```python
from build123d import *


with BuildPart() as part:
    # Sketch1 → Revolve1 (revolve)
    with BuildSketch(Plane(origin=(0, 0, 0), x_dir=(0, -1, 0), z_dir=(0, 0, -1)), mode=Mode.PRIVATE) as revolve1_sk:
        with BuildLine():
            Line((0, 1.5), (0, 12.78))
            Line((0, 12.78), (-0.18, 12.78))
            Line((-0.18, 12.78), (-0.18, 7.65))
            Line((-0.18, 7.65), (-0.5, 7.65))
            Line((-0.5, 7.65), (-0.5, 6.8))
            ThreePointArc((-0.5, 6.8), (-0.646446609, 6.446446609), (-1, 6.3))
            Line((-1, 6.3), (-3.7, 6.3))
            Line((-3.7, 6.3), (-4.2, 5.8))
            Line((-4.2, 5.8), (-4.2, 5.1))
            Line((-4.2, 5.1), (-5.4, 5.1))
            Line((-5.4, 5.1), (-5.9, 4.6))
            Line((-5.9, 4.6), (-5.9, 2))
            Line((-5.9, 2), (-5.4, 1.5))
            Line((-5.4, 1.5), (0, 1.5))
        make_face()
    revolve(revolve1_sk.sketch.rotate(Axis((0, 0, 0), (0, 1, 0)), 180), axis=Axis((0, 0, 0), (0, 1, 0)))


solid = part.part
```
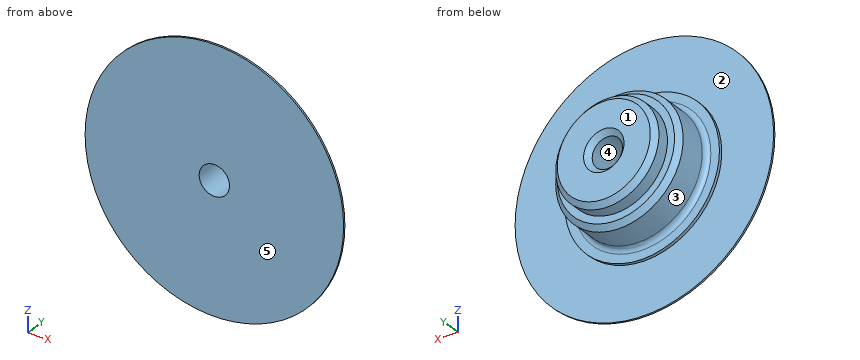
Could you check a few things on this model? Use its own coordinates, in mm. Face numbers are marked on the shaded views. A direction names the side the tool comes from. Round coordinates to 2 decimals unless told otherwise and drop trailing zeros. Order: outer loops, then holes, each group sorted by start corner. A loop starts at its lowest first (then second) coordinate and runs counter-clockwise, first axis right, second up. Notation, with made-up numbers: M 77.5,4 L 135.5,4 A23 cw 135.5,16 Z; hole C -34,-3.5 d10. An arc over 180 degrees is marked long. One line per question, with ' | ' between items. Start each with the question number.
(1) Suppose I cut it at B-B on x = 0. List the corners of the cut face in (y, z) for me, then the cut area to 3 significant figures.
(2) For P1, Ø1, axis at y = 1.5, z = -4.5, coming from the +X side; P2, Ø7.5, axis at x = -3.5, z = 3.5, coming from the +Y side; P3, Ø1, axis at y = 0.5, z = -2, coming from the -X side, each with a flat end and sliding along its axis, tell me the tip position at first contact or that it passes through.
(3) Suppose I cut it at C-C on y = 1.45. List the corners of the cut face in (x, z) for me.
(4) Suppose I cut it at D-D on z = -9.25. List the corners of the cut face in (x, y) for me.
(5) Suppose I cut it at A-A on z = 0. List the corners of the cut face in (x, y) for me.
(6) For the marked faces 1 and 2, which set-ups out of +Z, -Z, +X, -X, +Y, -Y let a thin tool reach every point of the face, with its end or its side?
(7) Thinking about a two-plate mould opening in X: for the marked faces 3, 4 and 5, which applies, +X half, -X half, draft (parallel to the pull), parting line (faces both ways), or undercut?
(8) Please list where these lines run through material, in increasing order: line 1 along Z through (x, y) = (0, 2.1); line 2 along Y through (x, z) = (8.75, -3.5); line 3 along Z through (x, y) = (1, 5.5).
Geometry results:
1) outline: M 0,-12.78 L 0.18,-12.78 L 0.18,-7.65 L 0.5,-7.65 L 0.5,-6.8 A0.5 cw 1,-6.3 L 3.7,-6.3 L 4.2,-5.8 L 4.2,-5.1 L 5.4,-5.1 L 5.9,-4.6 L 5.9,-2 L 5.4,-1.5 L 0,-1.5 Z; M 0,1.5 L 5.4,1.5 L 5.9,2 L 5.9,4.6 L 5.4,5.1 L 4.2,5.1 L 4.2,5.8 L 3.7,6.3 L 1,6.3 A0.5 cw 0.5,6.8 L 0.5,7.65 L 0.18,7.65 L 0.18,12.78 L 0,12.78 Z | area: 55.1 mm²
2) P1: x = 4.87 | P2: y = 5.9 | P3: x = -12.68
3) outline: C 0,0 d12.6; hole C 0,0 d3
4) outline: M -8.82,0 L 8.82,0 L 8.82,0.18 L -8.82,0.18 Z
5) outline: M -12.78,0 L -1.5,0 L -1.5,5.4 L -2,5.9 L -4.6,5.9 L -5.1,5.4 L -5.1,4.2 L -5.8,4.2 L -6.3,3.7 L -6.3,1 A0.5 cw -6.8,0.5 L -7.65,0.5 L -7.65,0.18 L -12.78,0.18 Z; M 1.5,0 L 12.78,0 L 12.78,0.18 L 7.65,0.18 L 7.65,0.5 L 6.8,0.5 A0.5 cw 6.3,1 L 6.3,3.7 L 5.8,4.2 L 5.1,4.2 L 5.1,5.4 L 4.6,5.9 L 2,5.9 L 1.5,5.4 Z
6) face 1: +Z, -Z, +X, -X, +Y | face 2: +Y
7) face 3: parting line | face 4: undercut | face 5: draft
8) line 1: -6.3 to -1.5, 1.5 to 6.3 | line 2: 0 to 0.18 | line 3: -4.9 to -1.25, 1.25 to 4.9
